from build123d import *

# Parameters (mm, degrees)
SKETCH1_R           = 1.125
SKETCH1_W           = 22.98
SKETCH1_H           = 12.65
BOSS_EXTRUDE1_DEPTH = 5
SKETCH1_3_R         = 2.5
BOSS_EXTRUDE2_DEPTH = 9
SKETCH1_4_R         = 2.5
BOSS_EXTRUDE3_DEPTH = 15


with BuildPart() as part:
    # Sketch1 → Boss-Extrude1 (new body)
    with BuildSketch(Plane(origin=(0, 0, 0), x_dir=(1, 0, 0), z_dir=(0, 1, 0))):
        with BuildLine():
            Line((32.5, 1.402234115), (32.5, 18.1625))
            ThreePointArc((32.5, 18.1625), (29.571067812, 25.233567812), (22.5, 28.1625))
            Line((22.5, 28.1625), (-22.5, 28.1625))
            ThreePointArc((-22.5, 28.1625), (-29.571067812, 25.233567812), (-32.5, 18.1625))
            Line((-32.5, 18.1625), (-32.5, 1.402234115))
            ThreePointArc((-32.5, 1.402234115), (-32.446161571, 0.670465224), (-32.285805716, -0.045544752))
            Line((-32.285805716, -0.045544752), (-24.854600808, -24.610278867))
            ThreePointArc((-24.854600808, -24.610278867), (-23.048820734, -27.177403133), (-20.068795092, -28.1625))
            Line((-20.068795092, -28.1625), (20.068795092, -28.1625))
            ThreePointArc((20.068795092, -28.1625), (23.048820734, -27.177403133), (24.854600808, -24.610278867))
            Line((24.854600808, -24.610278867), (32.285805716, -0.045544752))
            ThreePointArc((32.285805716, -0.045544752), (32.446161571, 0.670465224), (32.5, 1.402234115))
        make_face()
        with Locations(Location((-13.78, -11.8375, 0), (0, 0, 270))):
            Circle(SKETCH1_R, mode=Mode.SUBTRACT)
        with Locations(Location((13.78, -11.8375, 0), (0, 0, 270))):
            Circle(SKETCH1_R, mode=Mode.SUBTRACT)
        with BuildLine():
            Line((15, 18.1625), (-15, 18.1625))
            ThreePointArc((-15, 18.1625), (-22.5, 10.6625), (-15, 3.1625))
            Line((-15, 3.1625), (15, 3.1625))
            ThreePointArc((15, 3.1625), (22.5, 10.6625), (15, 18.1625))
        make_face(mode=Mode.SUBTRACT)
        with Locations((0, -11.8375)):
            Rectangle(SKETCH1_W, SKETCH1_H, mode=Mode.SUBTRACT)
    extrude(amount=BOSS_EXTRUDE1_DEPTH)

    # Sketch1_3 → Boss-Extrude2 (add)
    with BuildSketch(Plane(origin=(0, 0, 0), x_dir=(1, 0, 0), z_dir=(0, 1, 0))):
        with BuildLine():
            ThreePointArc((15, 18.1625), (22.5, 10.6625), (15, 3.1625))
            Line((15, 3.1625), (-15, 3.1625))
            ThreePointArc((-15, 3.1625), (-22.5, 10.6625), (-15, 18.1625))
            Line((-15, 18.1625), (15, 18.1625))
        make_face()
        with Locations(Location((-15, 10.6625, 0), (0, 0, 270))):
            Circle(SKETCH1_3_R, mode=Mode.SUBTRACT)
        with Locations(Location((15, 10.6625, 0), (0, 0, 270))):
            Circle(SKETCH1_3_R, mode=Mode.SUBTRACT)
    extrude(amount=BOSS_EXTRUDE2_DEPTH)

    # Sketch1_4 → Boss-Extrude3 (add)
    with BuildSketch(Plane(origin=(0, 0, 0), x_dir=(1, 0, 0), z_dir=(0, 1, 0))):
        with Locations(Location((15, 10.6625, 0), (0, 0, 270))):
            Circle(SKETCH1_4_R)
        with Locations(Location((-15, 10.6625, 0), (0, 0, 270))):
            Circle(SKETCH1_4_R)
    extrude(amount=BOSS_EXTRUDE3_DEPTH)


solid = part.part
Model file for the job. Use its own axes, mm. A direction names the side the tool comes from. Give positions to 0.01 mm unless a question says otherwise; leave off trailing zeros. Order: outer loops, then holes, each group sorted by start corner. A loop starts at its lowest first (then second) coordinate and runs counter-clockwise, first axis right, second up. Notation, with made-up numbers: M -1,-12.75 L 12,-12.75 A17 cw 12,13.25 Z; hole C 63.25,36 d9. An arc over 180 degrees is marked long. Put each result on its own line as item: value. Start each with the question number.
(1) Pull direction Z, two halves, no side cores. Call faces 6 (the face through (-23.085, 2.465, 27.151)), 7 (the face through (0, 2, -28.162)), 8 (the face through (11.49, 2, 12)): released by +Z, released by -Z, zero draft, split by the parting line, or undercut.
(2) Band-saw the part on D-D on z = 1. Give the cut face in (x, y), then the cut area to 3 significant figures.
(3) Tool access for faces 1 (the face through (12.78, 11.96, -9.51)), 2 (the face through (0, 7, -3.162)), 3 (the face through (0, 2, 5.512)), 4 (the face through (-22.5, 7, -10.5)), 5 (the face through (0, 7, -18.162)): list every direction of +Z, -Z, +X, -X, +Y, -Y with a clear straight run to the whole face (end or side of a thin tool).
(4) Band-saw the part on B-B on x = 18.5. Give the cut face in (y, z).
(5) Pin check, flat tips, straight feed: pin 1 Ø1.2 at (x, y) = (-1, 6.5) entering from -Z; pin 2 Ø5 at (y, z) = (6.5, -20.5) entering from -X; pin 3 Ø3 at (x, y) = (3.5, 7) entering from +Z. Stop position of each tip, or through.
(6) Band-saw the part on C-C on z = 20.5. Give the cut face in (x, y), then the cut area to 3 significant figures.
(7) Drill centre lines: L1, parallel to Z at x = -8, y = 4.75; L2, parallel to Y at x = 16, z = 14.5; L3, parallel to Y at x = -8.5, z = -12.5. Where is each one in solid material? Low to high. Write a range as [from, to].
(8) Band-saw the part on A-A on x = -4. Give the cut face in (y, z).
Results below:
1. face 6: released by +Z
1. face 7: released by -Z
1. face 8: undercut
2. outline: M -32,0 L 32,0 L 32,5 L -32,5 Z
2. area: 320 mm2
3. face 1: +Y
3. face 2: +Z, +X, -X, +Y
3. face 3: +Y, -Y
3. face 4: -X, +Y
3. face 5: -Z, +X, -X, +Y
4. outline: M 0,-28.16 L 5,-28.16 L 5,-17.3 L 9,-17.3 L 9,-4.03 L 5,-4.03 L 5,28.16 L 0,28.16 Z
5. pin 1: stops at z = -18.16
5. pin 2: stops at x = -32.49
5. pin 3: stops at z = -3.16
6. outline: M -26.1,0 L 26.1,0 L 26.1,5 L -26.1,5 Z
6. area: 261 mm2
7. L1: z = [-28.16, 5.51], [18.16, 28.16]
7. L2: y = [0, 5]
7. L3: y = [0, 9]
8. outline: M 0,-28.16 L 5,-28.16 L 5,-18.16 L 9,-18.16 L 9,-3.16 L 5,-3.16 L 5,5.51 L 0,5.51 Z; M 0,18.16 L 5,18.16 L 5,28.16 L 0,28.16 Z
